from build123d import *

# Parameters (mm, degrees)
F0_W     = 76.2
F0_H     = 106.4723501976
F1_DEPTH = 5.207
F2_W     = 20.828
F2_H     = 7.0416366247
F3_DEPTH = 5.207


with BuildPart() as f1:
    # F0 (on Front) → F1 (new body)
    with BuildSketch(Plane.XZ):
        Rectangle(F0_W, F0_H)
    extrude(amount=F1_DEPTH)

    # F2 (on face) → F3 (cut, through all)
    with BuildSketch(Plane(origin=(0, 0, 0), x_dir=(-1, 0, 0), z_dir=(0, 1, 0))):
        with Locations((27.686, -49.7153567864)):
            Rectangle(F2_W, F2_H)
        with Locations((-27.686, -49.7153567864)):
            Rectangle(F2_W, F2_H)
    extrude(amount=-F3_DEPTH, mode=Mode.SUBTRACT)


solid = f1.part
Geometry: final body of the model. Coordinates: model frame, mm. A direction names the side the tool comes from. Coordinates: 2 decimals unless noted, no trailing zeros. Loops run counter-clockwise (first coordinate to the right, second up) from the corner with the lowest first, then second, coordinate; pieces in that order, holes last. Notation, with made-up numbers: M 88.25,35.5 L 131.25,35.5 A22 cw 131.25,48.5 Z; hole C -29.75,2 d6. An arc over 180 degrees is marked long. One line per item, written item: value. Start each with the question number.
1) Cut plane A-A (y = -2.8). Return loops of the section in (x, z), then the cut area to 3 significant figures.
2) Pin query (flat end, axial travel): P1, Ø2.5, axis at y = -3.5, z = -49.5, coming from the +X side; P2, Ø2.5, axis at y = -2.5, z = -49, coming from the -X side. Return the tip coordinate at first contact, or that it passes through.
3) Material intervals for L1, parallel to Z at x = 30.5, y = -4.5; L2, parallel to X at y = -1.4, z = -46.5, sorted ascending. Write a range as from..to.
4) Reachability of faces 1 (the flat face through (-17.272, -3, -50)), 2 (the flat face through (-1, -3, 53.236)), 3 (the flat face through (17.272, -3, -50)) from +Z, -Z, +X, -X, +Y, -Y: full face, straight path, thin tool, end or side. Return the list, or none.
5) Cut plane B-B (x = -31). Return loops of the section in (y, z).
Evaluation:
1. outline: M -38.1,-46.19 L -17.27,-46.19 L -17.27,-53.24 L 17.27,-53.24 L 17.27,-46.19 L 38.1,-46.19 L 38.1,53.24 L -38.1,53.24 Z
1. area: 7,820 mm^2
2. P1: x = 17.27
2. P2: x = -17.27
3. L1: -46.19..53.24
3. L2: -17.27..17.27
4. face 1: -Z, -X, +Y, -Y
4. face 2: +Z, +X, -X, +Y, -Y
4. face 3: -Z, +X, +Y, -Y
5. outline: M -5.21,-46.19 L 0,-46.19 L 0,53.24 L -5.21,53.24 Z
